Verification items for the finished model (mm, model axes). Face numbers are marked on the shaded views. A direction names the side the tool comes from. Give positions to 0.01 mm unless a question says otherwise; leave off trailing zeros. Loops run counter-clockwise (first coordinate to the right, second up) from the corner with the lowest first, then second, coordinate; pieces in that order, holes last. Notation, with made-up numbers: (15, 31) -> (71, 31) arc R21 cw to (71, 62) -> close; hole circle Ø4 at (58.25, -30.5). An arc over 180 degrees is marked (long way). Answer in a Markdown table with one row per item. Add a question column.
Q1. Section check D-D on x = 27.5. Enter the section's corners in (y, z), and give its area (3 significant figures).
Q2. Section check A-A on y = 26. Enter the section's corners in (x, z), and give its area (3 significant figures).
Q3. Material ranges on probe 1 along Y at (x, z) = (28.5, 30); probe 2 along Z at (x, y) = (23, 28.5); probe 3 along X at (y, z) = (39, 10.5), recorded low to high.
Q4. Section check C-C on z = 35.5. Enter the section's corners in (x, y).
Q5. Gauge pin test, flat ends, axial feed: P1, Ø1.5, axis at y = 22.5, z = 10.5, coming from the -X side; P2, Ø20.5, axis at x = 29.5, y = 22, coming from the +Z side; P3, Ø22, axis at y = 28.5, z = 24.5, coming from the -X side. Record the tip position at first contact, or that the pin passes through.
Q6. Set-up check for the marked faces 1 and 2: record each of +Z, -Z, +X, -X, +Y, -Y from which the full face is reachable in a straight line by a thin tool's end or side.
Q7. Release check for a two-part mould opening along Y. For the marked faces 3, 4 and 5 record: pulls with the +Y half, pulls with the -Y half, needs draft (parallel to the pull), parting line crosses it, or undercut.
Q8. Section check B-B on y = 9.5. Enter the section's corners in (x, z), and give its area (3 significant figures).
```python
from build123d import *

# Parameters (mm, degrees)
F0_W     = 76.2
F0_H     = 50.8
F1_DEPTH = 38.1
F3_DEPTH = 50.8
F4_W     = 44.3217208988
F4_H     = 40.64
F5_DEPTH = 27.8086844974
F6_R     = 6.35
F7_DEPTH = 13.4962615407
F8_R     = 6.35
F9_DEPTH = 13.4962615407


with BuildPart() as f1:
    # F0 (on Top) → F1 (new body)
    with BuildSketch(Plane.XY):
        with Locations((38.1, 25.4)):
            Rectangle(F0_W, F0_H)
    extrude(amount=F1_DEPTH)

    # F2 (on face) → F3 (cut, through all)
    with BuildSketch(Plane.XZ):
        Polygon((0, 38.1), (0, 8.26475929), (10.8591395506, 38.1), align=None)
        Polygon((76.2, 38.1), (65.3408604494, 38.1), (76.2, 8.26475929), align=None)
    extrude(amount=-F3_DEPTH, mode=Mode.SUBTRACT)

    # F4 (on face) → F5 (cut, through all)
    with BuildSketch(Plane.XY.offset(38.1)):
        with Locations((38.1, 25.4)):
            Rectangle(F4_W, F4_H)
    extrude(amount=-F5_DEPTH, mode=Mode.SUBTRACT)

    # F6 (on face) → F7 (cut, through all)
    with BuildSketch(Plane(origin=(-2.6562424343, 0, 0.9667931811), x_dir=(0, -1, 0), z_dir=(-0.9396926208, 0, 0.3420201433))):
        with Locations((-25.4, 23.6413333174)):
            Circle(F6_R)
    extrude(amount=-F7_DEPTH, mode=Mode.SUBTRACT)

    # F8 (on face) → F9 (cut, through all)
    with BuildSketch(Plane(origin=(69.9425357172, 0, 25.4570011102), x_dir=(0, 1, 0), z_dir=(0.9396926208, 0, 0.3420201433))):
        with Locations((25.4, -2.420601604)):
            Circle(F8_R)
    extrude(amount=-F9_DEPTH, mode=Mode.SUBTRACT)


solid = f1.part
```
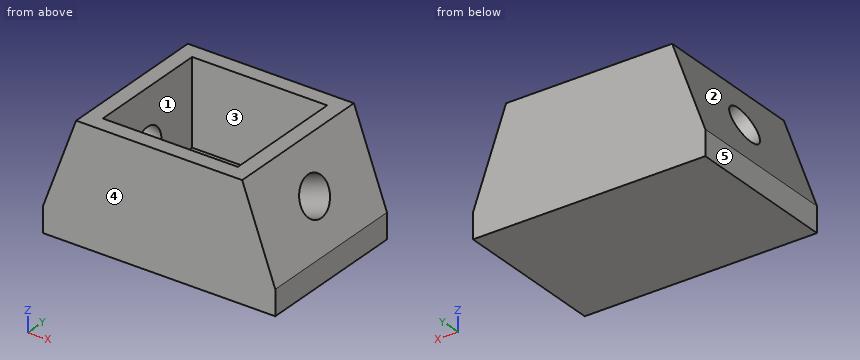
Taken from the geometry:
| question | item | result |
|---|---|---|
| 1 | outline | (0, 0) -> (50.8, 0) -> (50.8, 38.1) -> (45.72, 38.1) -> (45.72, 10.29) -> (5.08, 10.29) -> (5.08, 38.1) -> (0, 38.1) -> close |
| 1 | area | 805 mm² |
| 2 | outline | (0, 0) -> (76.2, 0) -> (76.2, 8.26) -> (72.93, 17.24) -> (60.26, 12.63) -> (60.26, 10.29) -> (15.94, 10.29) -> (15.94, 12.63) -> (3.27, 17.24) -> (0, 8.26) -> close; (7.59, 29.12) -> (15.94, 26.08) -> (15.94, 38.1) -> (10.86, 38.1) -> close; (60.26, 26.08) -> (68.61, 29.12) -> (65.34, 38.1) -> (60.26, 38.1) -> close |
| 2 | area | 1,060 mm² |
| 3 | probe 1 | y = 0 to 5.08, 45.72 to 50.8 |
| 3 | probe 2 | z = 0 to 10.29 |
| 3 | probe 3 | x = 0.81 to 15.94, 60.26 to 75.39 |
| 4 | outline | (9.91, 0) -> (66.29, 0) -> (66.29, 50.8) -> (9.91, 50.8) -> close; hole (15.94, 5.08) -> (60.26, 5.08) -> (60.26, 45.72) -> (15.94, 45.72) -> close |
| 5 | P1 | stops at x = 0.54 |
| 5 | P2 | stops at z = 10.29 |
| 5 | P3 | stops at x = 1.91 |
| 6 | face 1 | +Z |
| 6 | face 2 | +Z, -X, +Y, -Y |
| 7 | face 3 | undercut |
| 7 | face 4 | pulls with the -Y half |
| 7 | face 5 | needs draft |
| 8 | outline | (0, 0) -> (76.2, 0) -> (76.2, 8.26) -> (65.34, 38.1) -> (60.26, 38.1) -> (60.26, 10.29) -> (15.94, 10.29) -> (15.94, 38.1) -> (10.86, 38.1) -> (0, 8.26) -> close |
| 8 | area | 1,350 mm² |
